Part print with two shaded views. Sizes in mm from the minimum x, y, z corner. Round coordinates to 2 decimals unless told otherwise and drop trailing zeros. Write each loop counter-clockwise with the first axis right and the second up, starting at its lowest first coordinate (ties: lowest second). Pieces come first, ordered by that corner, then holes. Notation, with made-up numbers: (44.25, -29.75) - (100.25, -29.75) arc R28 ccw to (100.25, -10.75) - close; hole circle Ø11 at (5.5, 86.25). An arc over 180 degrees is marked (long way). Answer as a JSON object with one key per item and string values. Group by question number.
Item 1: Slice it at A-A, the plane y = 57.15. List the corners of the cut face in (x, z).
Item 2: Flat gauge pin, fed straight in: pin 1 (1 mm diameter, centred on x = 0.5, y = 67, fed in from +Z). Where does the tip first touch, or does it go through?
Item 3: Slice it at B-B, the plane z = 10.5. List the corners of the cut face in (x, y).
Item 4: Probe line 1 (Y direction, x = 2.8, z = 20.25); line 2 (Y direction, x = 0.95, z = 3); line 3 (Z direction, x = 2.85, y = 29). List the from-to ranges inside material, lowest first. Write a range as from..to.
Item 5: Slice it at C-C, the plane x = 1.05. Give the number of separate pieces and of enclosed holes in the cut face, then the cut area to 3 significant figures.
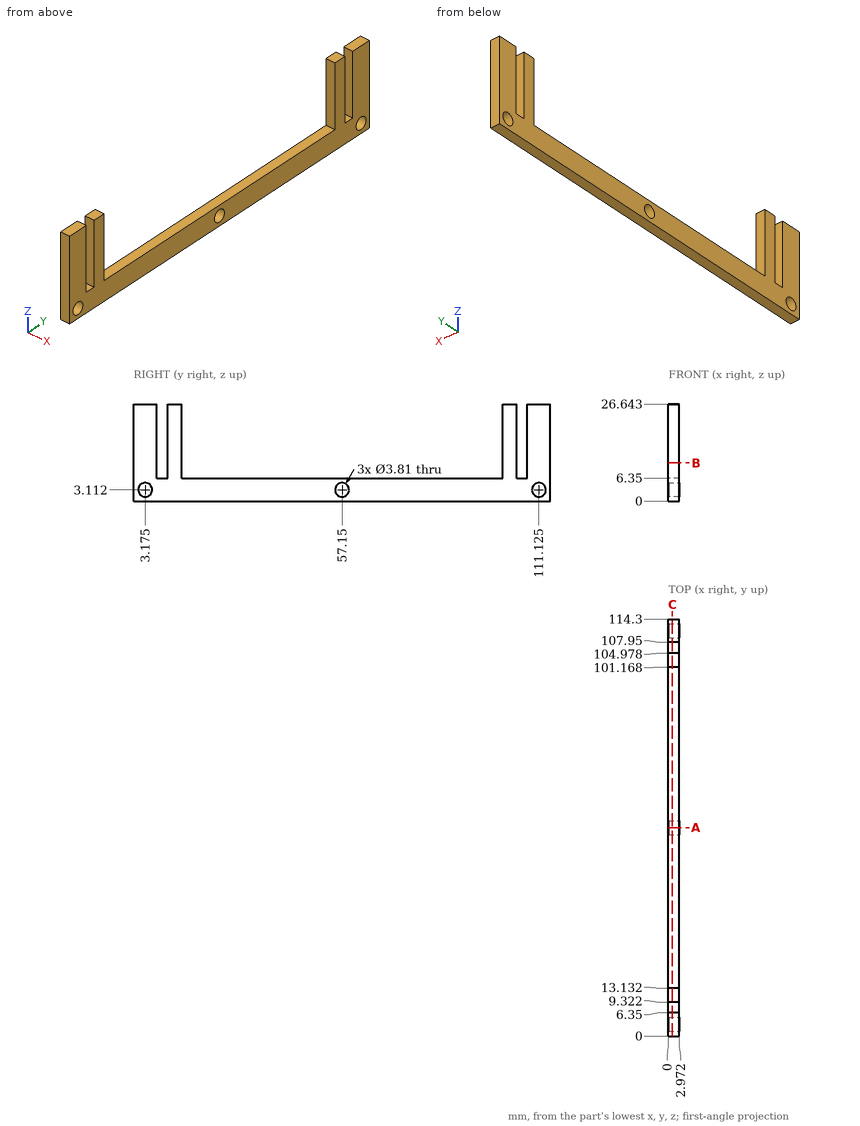
Geometry says:
{
 "1": {"outline": "(0, 0) - (2.97, 0) - (2.97, 1.21) - (0, 1.21) - close; (0, 5.02) - (2.97, 5.02) - (2.97, 6.35) - (0, 6.35) - close"},
 "2": {"pin 1": "stops at z = 6.35"},
 "3": {"outline": "(0, 0) - (2.97, 0) - (2.97, 6.35) - (0, 6.35) - close; (0, 9.32) - (2.97, 9.32) - (2.97, 13.13) - (0, 13.13) - close; (0, 101.17) - (2.97, 101.17) - (2.97, 104.98) - (0, 104.98) - close; (0, 107.95) - (2.97, 107.95) - (2.97, 114.3) - (0, 114.3) - close"},
 "4": {"line 1": "y = 0..6.35, 9.32..13.13, 101.17..104.98, 107.95..114.3", "line 2": "y = 0..1.27, 5.08..55.25, 59.05..109.22, 113.03..114.3", "line 3": "z = 0..6.35"},
 "5": {"separate pieces": "1", "enclosed holes": "3", "area": "1,100 mm^2"}
}
